Design review of the part shown in the three views and the two pictorial views. Dimensions are in mm from the part's minimum x, y and z. A direction names the side the tool comes from. Coordinates: 2 decimals unless noted, no trailing zeros. Order: outer loops, then holes, each group sorted by start corner. A loop starts at its lowest first (then second) coordinate and runs counter-clockwise, first axis right, second up. Notation, with made-up numbers: (71, 75) -> (99, 75) arc R26 ccw to (99, 100) -> close; hole circle Ø11 at (-27.75, 85). An arc over 180 degrees is marked (long way). Answer as a JSON object with one key per item and string values. Group by question number.
1) Add section D-D, the plane x = 3. Write out the cut boundary in (y, z), then the cut area to 3 significant figures.
2) Add section C-C, the plane x = 10. Write out the cut boundary in (y, z), then the cut area to 3 significant figures.
3) Add section A-A, the plane y = 12.7. Write out the cut boundary in (x, z).
4) Machinability: for the marked faces 1, 2 and 3, which of the approach directions +Z, -Z, +X, -X, +Y, -Y give a long, thin tool a straight path to every point of the face, cutting with its end or side? Answer none if there is none.
5) For pin 1 (3 mm diameter, centred on x = 19, y = 4.5, fed in from -Z); pin 2 (1 mm diameter, centred on x = 36, z = 16, fed in from -Y); pin 3 (5 mm diameter, centred on x = 7.5, y = 22.5, fed in from -Z); pin 4 (2 mm diameter, centred on x = 6.5, y = 13, fed in from +Z), all flat-tipped, find the tip position at first contact; note any pin that passes through.
6) Wall thickness on L1, parallel to X at y = 22.25, z = 16.75; L2, parallel to Y at x = 29, z = 19.75; L3, parallel to Y at x = 34, z = 2.5: over which ranges is each line inside the solid? List them lowest first.
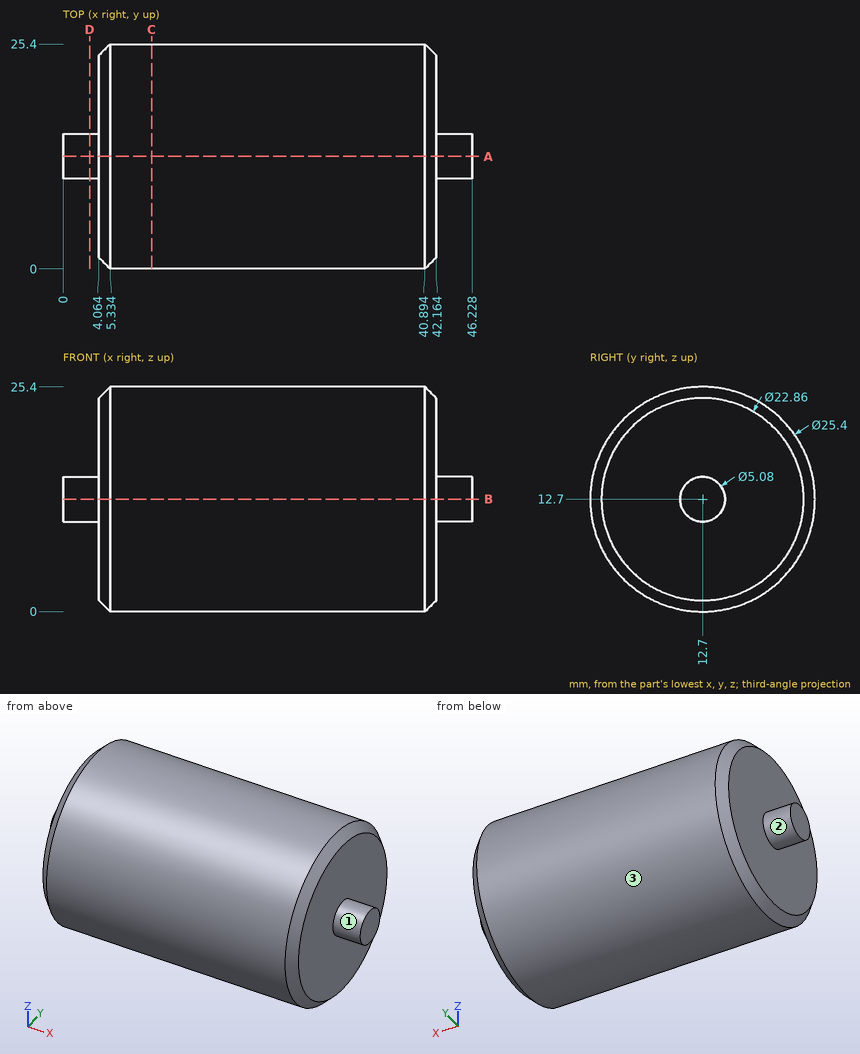
Output values:
{
 "1": {"outline": "circle Ø5.08 at (12.7, 12.7)", "area": "20.3 mm²"},
 "2": {"outline": "circle Ø25.4 at (12.7, 12.7)", "area": "507 mm²"},
 "3": {"outline": "(0, 10.16) -> (4.06, 10.16) -> (4.06, 1.27) -> (5.33, 0) -> (40.89, 0) -> (42.16, 1.27) -> (42.16, 10.16) -> (46.23, 10.16) -> (46.23, 15.24) -> (42.16, 15.24) -> (42.16, 24.13) -> (40.89, 25.4) -> (5.33, 25.4) -> (4.06, 24.13) -> (4.06, 15.24) -> (0, 15.24) -> close"},
 "4": {"face 1": "+X", "face 2": "-X", "face 3": "+X, -X"},
 "5": {"pin 1": "stops at z = 1.91", "pin 2": "stops at y = 0.31", "pin 3": "stops at z = 2.31", "pin 4": "stops at z = 25.4"},
 "6": {"L1": "x = 4.06 to 42.16", "L2": "y = 2.14 to 23.26", "L3": "y = 5.13 to 20.27"}
}
